```python
from build123d import *

# Parameters (mm, degrees)
SKETCH1_W          = 24.0665
SKETCH1_H          = 1.999996
SKETCH3_R          = 18.415
CUT_EXTRUDE1_DEPTH = 2.999996


with BuildPart() as part:
    # Sketch1 → Revolve1 (revolve)
    with BuildSketch(Plane.XY):
        with Locations((12.03325, 0)):
            Rectangle(SKETCH1_W, SKETCH1_H)
    revolve(axis=Axis((0, 0.999998, 0), (0, -1, 0)))

    # Sketch2 → Cut-Revolve1 (revolve, cut)
    with BuildSketch(Plane.XY):
        Polygon((-20.955, 0.635), (-20.955, 1.799850338), (-24.1554, 1.799850338), align=None)
        Polygon((-24.1554, -1.799850338), (-20.955, -0.635), (-20.955, -1.799850338), align=None)
    revolve(axis=Axis((0, 0, 0), (0, 1, 0)), mode=Mode.SUBTRACT)

    # Sketch3 → Cut-Extrude1 (cut, through all)
    with BuildSketch(Plane(origin=(0, 0.999998, 0), x_dir=(1, 0, 0), z_dir=(0, 1, 0))):
        Circle(SKETCH3_R)
    extrude(amount=-CUT_EXTRUDE1_DEPTH, mode=Mode.SUBTRACT)


solid = part.part
```
The listing builds one solid part. Answer for the finished solid, in the listing's coordinates (mm). Give positions to 0.01 mm unless a question says otherwise; leave off trailing zeros. Order: outer loops, then holes, each group sorted by start corner. A loop starts at its lowest first (then second) coordinate and runs counter-clockwise, first axis right, second up. Notation, with made-up numbers: (-25.75, -32.5) -> (8.25, -32.5) arc R23 ccw to (8.25, -10.5) -> close; hole circle Ø2 at (5, 0). An arc over 180 degrees is marked (long way). Write each question's results on one line, items separated by ' | '.
Q1. Straight lines are drawn through the part: probe 1 along Z at (x, y) = (0, -0.45) (1 decimal); probe 2 along Z at (x, y) = (-12.5, -0.35); probe 3 along X at (y, z) = (-0.05, 11.5). For each, find the intervals that lie inside material, in ascending order. Write a range as from..to.
Checked values:
probe 1: z = -24.1..-18.4, 18.4..24.1 | probe 2: z = -20.57..-13.52, 13.52..20.57 | probe 3: x = -21.14..-14.38, 14.38..21.14
Q2. The part is cut by section C-C, the plane y = -0.1. Give the vertices of the cut face in (x, z) (1 decimal).
Checked values:
outline: circle Ø48.1 at (0, 0); hole circle Ø36.8 at (0, 0)
Q3. This flat-tipped pin is pushed along its axis until it touches: P1, Ø1, axis at x = -7, y = 0, coming from the +Z side. Where does it stop, or does it pass through?
Checked values:
P1: stops at z = 23.17
Q4. Determine the mould class of faces 1 (the face through (-5.2, 0, -23.5)), 2 (the face through (0, -1, -19)), 3 (the face through (-14.61, 0.01, 11.21)) for opening direction X: pulls with the +X half, pulls with the -X half, needs draft (parallel to the pull), parting line crosses it, or undercut.
Checked values:
face 1: parting line crosses it | face 2: needs draft | face 3: undercut
